from build123d import *

# Parameters (mm, degrees)
F0_R          = 9.15
F1_DEPTH      = 30
F2_SIZE2      = 1
F2_SIZE       = 1
F5_DEPTH      = 3
F5_DEPTH_BACK = 8
F6_DEPTH      = 25
F6_DEPTH_BACK = 25


with BuildPart() as f1:
    # F0 (on Front) → F1 (new body)
    with BuildSketch(Plane.XZ):
        Circle(F0_R)
    extrude(amount=F1_DEPTH)

    # F2
    f2_edges = [f1.edges().sort_by_distance(p)[0] for p in [
        (-9.15, -30, 0),
    ]]
    chamfer(f2_edges, length=F2_SIZE, length2=F2_SIZE2)

    # F4 (on offset) → F5 (cut, two sides)
    with BuildSketch(Plane.XZ.offset(20)) as f5_sk:
        with BuildLine():
            Line((0, -4.4547727215), (-4.4547727215, 0))
            Line((-4.4547727215, 0), (-8.3019233801, -3.8471506587))
            ThreePointArc((-8.3019233801, -3.8471506587), (-6.4700270479, -6.4700270479), (-3.8471506587, -8.3019233801))
            Line((-3.8471506587, -8.3019233801), (0, -4.4547727215))
        make_face()
    extrude(amount=F5_DEPTH, mode=Mode.SUBTRACT)
    extrude(f5_sk.sketch, amount=-F5_DEPTH_BACK, mode=Mode.SUBTRACT)

    # F6 (cut, two sides): a face of the model
    f6_faces = [f1.faces().sort_by_distance(p)[0] for p in [
        (-6.3783480508, -17.5, -1.9235753293),
    ]]
    extrude(f6_faces, amount=-F6_DEPTH, mode=Mode.SUBTRACT)
    extrude(f6_faces, amount=F6_DEPTH_BACK, mode=Mode.SUBTRACT)


solid = f1.part
Build history of the part. All positions in model axes, mm. A direction names the side the tool comes from. Round coordinates to 2 decimals unless told otherwise and drop trailing zeros. Write each loop counter-clockwise with the first axis right and the second up, starting at its lowest first coordinate (ties: lowest second). Pieces come first, ordered by that corner, then holes. Notation, with made-up numbers: M 5,82 L 39,82 A15 cw 39,98 Z; hole C -1,-37 d6. An arc over 180 degrees is marked long. Answer in a Markdown table with one row per item.
1. Mould opens along Y. For faces 1 (the face through (-4, -12, -4)), 2 (the face through (0, 0, 0)), 3 (the face through (0, -30, 0)) say: +Y half, -Y half, draft (parallel to the pull), parting line (faces both ways), or undercut.
Geometry check:
| item | result |
|---|---|
| face 1 | undercut |
| face 2 | +Y half |
| face 3 | -Y half |
2. Probe L1, parallel to Y at x = -2, z = -7.5; L2, parallel to X at y = -2, z = -0.25; L3, parallel to X at y = -15.5, z = 7. List the from-to ranges inside material, lowest first. Write a range as [from, to].
Geometry check:
| item | result |
|---|---|
| L1 | [-30, -23], [-12, 0] |
| L2 | [-9.15, 9.15] |
| L3 | [-5.89, 5.89] |
3. Which spindle directions (+Z, -Z, +X, -X, +Y, -Y) get a long thin tool onto all of the face, cutting with end or side? Do faces 4 (the face through (-4, -23, -4)), 5 (the face through (4.919, -14.297, 7.715)). Say none if no direction does.
Geometry check:
| item | result |
|---|---|
| face 4 | -Z, -X |
| face 5 | +Y, -Y |
4. Saw through at A-A (y = -15.5). List the corners of the cut face in (x, z).
Geometry check:
| item | result |
|---|---|
| outline | M -8.3,3.85 L 3.85,-8.3 A9.15 ccw long Z |
5. Saw through at B-B (y = -2.5). List the corners of the cut face in (x, z).
Geometry check:
| item | result |
|---|---|
| outline | C 0,0 d18.3 |
6. Flat gauge pins, fed straight in: P1, Ø1.5, axis at x = 2, y = -3, coming from the +Z side; P2, Ø2, axis at y = -5, z = -5.5, coming from the +X side; P3, Ø1, axis at y = -3, z = 6, coming from the +X side. Where does each tip first touch, or does it go through?
Geometry check:
| item | result |
|---|---|
| P1 | z = 9.06 |
| P2 | x = 7.97 |
| P3 | x = 7.31 |
